Geometry check sheet. Reference: drawing and pictorial views, mm from the part's lowest x, y, z. A direction names the side the tool comes from. Give positions to 0.01 mm unless a question says otherwise; leave off trailing zeros. Write each loop counter-clockwise with the first axis right and the second up, starting at its lowest first coordinate (ties: lowest second). Pieces come first, ordered by that corner, then holes. Notation, with made-up numbers: (76, 15.25) -> (83, 15.25) arc R28 ccw to (83, 43.25) -> close; hole circle Ø3 at (-35, -8). An arc over 180 degrees is marked (long way). Answer as CSV lines item,"result".
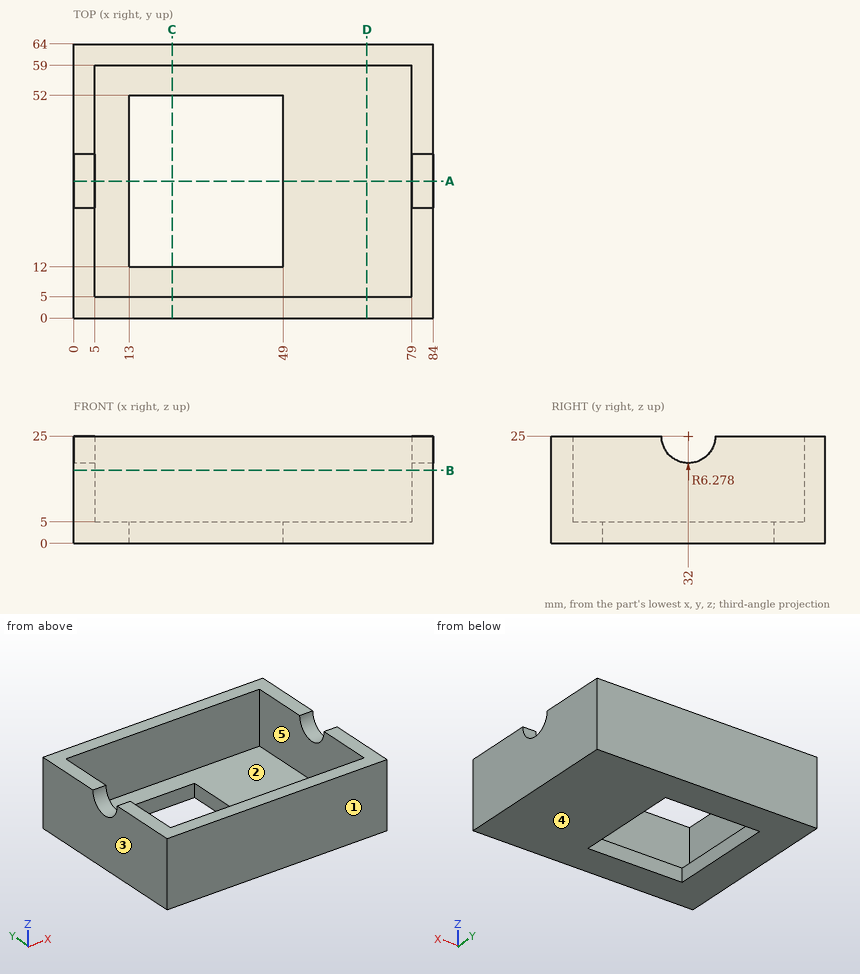
1) Draft check along X on the marked faces 3, 4 and 5. Enter one of: +X half, -X half, draft (parallel to the pull), parting line (faces both ways), or undercut.
Reported:
face 3,"-X half"
face 4,"draft"
face 5,"undercut"
2) Scan lines: line 1 along Y through (x, z) = (59, 13.75); line 2 along X through (y, z) = (11, 7.75); line 3 along Y through (x, z) = (33.5, 4.5). Record each from-to range of solid material in increasing order.
Reported:
line 1,"0 to 5, 59 to 64"
line 2,"0 to 5, 79 to 84"
line 3,"0 to 12, 52 to 64"
3) Section check C-C (x = 23). Record the boundary of the cut face in (y, z), and give its area (3 significant figures).
Reported:
outline,"(0, 0) -> (12, 0) -> (12, 5) -> (5, 5) -> (5, 25) -> (0, 25) -> close; (52, 0) -> (64, 0) -> (64, 25) -> (59, 25) -> (59, 5) -> (52, 5) -> close"
area,"320 mm²"
4) Section check B-B (z = 17). Record the boundary of the cut face in (x, y), and give its area (3 significant figures).
Reported:
outline,"(0, 0) -> (84, 0) -> (84, 64) -> (0, 64) -> close; hole (5, 5) -> (79, 5) -> (79, 59) -> (5, 59) -> close"
area,"1,380 mm²"
5) Section check A-A (y = 32). Record the boundary of the cut face in (x, z), and give its area (3 significant figures).
Reported:
outline,"(0, 0) -> (13, 0) -> (13, 5) -> (5, 5) -> (5, 18.72) -> (0, 18.72) -> close; (49, 0) -> (84, 0) -> (84, 18.72) -> (79, 18.72) -> (79, 5) -> (49, 5) -> close"
area,"377 mm²"
6) Tool access check on the marked faces 1 and 2. Record the directions out of +Z, -Z, +X, -X, +Y, -Y that give a thin tool (end or side, any length) a straight path to the whole face; none if there is none.
Reported:
face 1,"+Z, -Z, +X, -X, -Y"
face 2,"+Z"
7) Section check D-D (x = 68.5). Record the boundary of the cut face in (y, z), and give its area (3 significant figures).
Reported:
outline,"(0, 0) -> (64, 0) -> (64, 25) -> (59, 25) -> (59, 5) -> (5, 5) -> (5, 25) -> (0, 25) -> close"
area,"520 mm²"
8) Depth check by flat-ended pin: pin 1 (3 mm diameter, centred on x = 72.5, y = 26, fed in from +Z). Enter the tip coordinate at first touch or a pass-through.
Reported:
pin 1,"z = 5"
